Verification items for the finished model (mm, model axes). A direction names the side the tool comes from. Round coordinates to 2 decimals unless told otherwise and drop trailing zeros. Write each loop counter-clockwise with the first axis right and the second up, starting at its lowest first coordinate (ties: lowest second). Pieces come first, ordered by that corner, then holes. Notation, with made-up numbers: (18.5, 61.5) - (42.5, 61.5) arc R14 ccw to (42.5, 86.5) - close; hole circle Ø2 at (55.5, -22.5). An arc over 180 degrees is marked (long way). Write each question's results on one line, items separated by ' | '.
```python
from build123d import *

# Parameters (mm, degrees)
SKETCH_1_W           = 113
SKETCH_1_H           = 113
EXTRUDE_1_DEPTH      = 3
CUT_EXTRUDE_1_REACH  = 161.834
SKETCH_2_R           = 1.7
SKETCH_3_W           = 90
SKETCH_3_H           = 105
EXTRUDE_2_DEPTH      = 2
SKETCH_5_R           = 5
EXTRUDE_3_DEPTH      = 3
CUT_EXTRUDE_2_REACH  = 161.834
SKETCH_6_R           = 1.7
CUT_EXTRUDE_3_REACH  = 161.834
SKETCH_7_R           = 1.7
CUT_EXTRUDE_4_REACH  = 161.884
SKETCH_8_R           = 1.7
EXTRUDE_5_DEPTH      = 90
CUT_EXTRUDE_5_DEPTH  = 2
SKETCH_13_W          = 2
SKETCH_13_H          = 12
EXTRUDE_6_DEPTH      = 11.5
CUT_EXTRUDE_6_REACH  = 162.612
SKETCH_14_R          = 1.7
CUT_EXTRUDE_7_REACH  = 164.681
EXTRUDE_7_DEPTH      = 8.5
SKETCH_17_W          = 2
SKETCH_17_H          = 11.5
EXTRUDE_8_DEPTH      = 3
FILLET_1_R           = 1
CUT_EXTRUDE_8_DEPTH  = 163.681089759
SKETCH_20_W          = 113
SKETCH_20_H          = 12.124355653
CUT_EXTRUDE_9_DEPTH  = 1
CHAMFER_1_SIZE       = 1
SKETCH_21_W          = 7
SKETCH_21_H          = 13.5
CUT_EXTRUDE_10_DEPTH = 163.681089759
SKETCH_22_W          = 5
SKETCH_22_H          = 24
CUT_EXTRUDE_11_DEPTH = 163.681089759
SKETCH_23_W          = 2
SKETCH_23_H          = 19.464101615
CUT_EXTRUDE_12_DEPTH = 2
CHAMFER_2_SIZE       = 2
SKETCH_24_W          = 0.692820323
SKETCH_24_H          = 0.4
CUT_EXTRUDE_13_DEPTH = 95.5
SKETCH_25_W          = 0.692820323
SKETCH_25_H          = 0.4
CUT_EXTRUDE_14_DEPTH = 5.5
SKETCH_26_W          = 0.692820323
SKETCH_26_H          = 0.4
CUT_EXTRUDE_15_DEPTH = 7.5
SKETCH_27_W          = 113
SKETCH_27_H          = 105.875644347
CUT_EXTRUDE_16_DEPTH = 163.339889035
SKETCH_29_W          = 10
SKETCH_29_H          = 5
CUT_EXTRUDE_17_DEPTH = 163.185818036
SKETCH_30_W          = 10
SKETCH_30_H          = 2
CUT_EXTRUDE_18_DEPTH = 37
SKETCH_31_W          = 10
SKETCH_31_H          = 27
EXTRUDE_9_DEPTH      = 1


with BuildPart() as part:
    # 草图1 → 凸台-拉伸1 (new body)
    with BuildSketch(Plane(origin=(0, 0, 0), x_dir=(1, 0, 0), z_dir=(0, 1, 0))):
        with Locations((56.5, 56.5)):
            Rectangle(SKETCH_1_W, SKETCH_1_H)
    extrude(amount=EXTRUDE_1_DEPTH)

    # 草图2 → 切除-拉伸1 (cut, up to next)
    with BuildSketch(Plane(origin=(0, 3, 0), x_dir=(1, 0, 0), z_dir=(0, 1, 0)), mode=Mode.PRIVATE) as cut_extrude_1_sk1:
        with Locations(Location((108.5, 69.95, 0), (0, 0, 270))):
            Circle(SKETCH_2_R)
    cut_extrude_1_tool1 = extrude(cut_extrude_1_sk1.sketch, amount=-CUT_EXTRUDE_1_REACH, mode=Mode.PRIVATE) & part.part
    # 草图2 → 切除-拉伸1 (cut, up to next)
    with BuildSketch(Plane(origin=(0, 3, 0), x_dir=(1, 0, 0), z_dir=(0, 1, 0)), mode=Mode.PRIVATE) as cut_extrude_1_sk2:
        with Locations(Location((108.5, 47.45, 0), (0, 0, 270))):
            Circle(SKETCH_2_R)
    cut_extrude_1_tool2 = extrude(cut_extrude_1_sk2.sketch, amount=-CUT_EXTRUDE_1_REACH, mode=Mode.PRIVATE) & part.part
    # 草图2 → 切除-拉伸1 (cut, up to next)
    with BuildSketch(Plane(origin=(0, 3, 0), x_dir=(1, 0, 0), z_dir=(0, 1, 0)), mode=Mode.PRIVATE) as cut_extrude_1_sk3:
        with Locations(Location((106, 30.4, 0), (0, 0, 270))):
            Circle(SKETCH_2_R)
    cut_extrude_1_tool3 = extrude(cut_extrude_1_sk3.sketch, amount=-CUT_EXTRUDE_1_REACH, mode=Mode.PRIVATE) & part.part
    # 草图2 → 切除-拉伸1 (cut, up to next)
    with BuildSketch(Plane(origin=(0, 3, 0), x_dir=(1, 0, 0), z_dir=(0, 1, 0)), mode=Mode.PRIVATE) as cut_extrude_1_sk4:
        with Locations(Location((106, 10.4, 0), (0, 0, 270))):
            Circle(SKETCH_2_R)
    cut_extrude_1_tool4 = extrude(cut_extrude_1_sk4.sketch, amount=-CUT_EXTRUDE_1_REACH, mode=Mode.PRIVATE) & part.part
    add(cut_extrude_1_tool1.solids().sort_by_distance((108.5, 3, -69.95))[0], mode=Mode.SUBTRACT)
    add(cut_extrude_1_tool2.solids().sort_by_distance((108.5, 3, -47.45))[0], mode=Mode.SUBTRACT)
    add(cut_extrude_1_tool3.solids().sort_by_distance((106, 3, -30.4))[0], mode=Mode.SUBTRACT)
    add(cut_extrude_1_tool4.solids().sort_by_distance((106, 3, -10.4))[0], mode=Mode.SUBTRACT)

    # 草图3 → 凸台-拉伸2 (add)
    with BuildSketch(Plane(origin=(0, 0, 0), x_dir=(1, 0, 0), z_dir=(0, 1, 0))):
        with Locations((55.5, 60.5)):
            Rectangle(SKETCH_3_W, SKETCH_3_H)
    extrude(amount=-EXTRUDE_2_DEPTH)

    # 草图5 → 凸台-拉伸3 (add)
    with BuildSketch(Plane.XZ):
        with Locations((79.5, -1)):
            Circle(SKETCH_5_R)
        with Locations((31.5, -1)):
            Circle(SKETCH_5_R)
    extrude(amount=-EXTRUDE_3_DEPTH)

    # 草图6 → 切除-拉伸2 (cut, up to next)
    with BuildSketch(Plane.XZ, mode=Mode.PRIVATE) as cut_extrude_2_sk1:
        with Locations(Location((31.5, -1, 0), (0, 0, 270))):
            Circle(SKETCH_6_R)
    cut_extrude_2_tool1 = extrude(cut_extrude_2_sk1.sketch, amount=-CUT_EXTRUDE_2_REACH, mode=Mode.PRIVATE) & part.part
    # 草图6 → 切除-拉伸2 (cut, up to next)
    with BuildSketch(Plane.XZ, mode=Mode.PRIVATE) as cut_extrude_2_sk2:
        with Locations(Location((79.5, -1, 0), (0, 0, 270))):
            Circle(SKETCH_6_R)
    cut_extrude_2_tool2 = extrude(cut_extrude_2_sk2.sketch, amount=-CUT_EXTRUDE_2_REACH, mode=Mode.PRIVATE) & part.part
    add(cut_extrude_2_tool1.solids().sort_by_distance((31.5, 0, -1))[0], mode=Mode.SUBTRACT)
    add(cut_extrude_2_tool2.solids().sort_by_distance((79.5, 0, -1))[0], mode=Mode.SUBTRACT)

    # 草图7 → 切除-拉伸3 (cut, up to next)
    with BuildSketch(Plane.XZ, mode=Mode.PRIVATE) as cut_extrude_3_sk1:
        with Locations(Location((5, -10.4, 0), (0, 0, 270))):
            Circle(SKETCH_7_R)
    cut_extrude_3_tool1 = extrude(cut_extrude_3_sk1.sketch, amount=-CUT_EXTRUDE_3_REACH, mode=Mode.PRIVATE) & part.part
    # 草图7 → 切除-拉伸3 (cut, up to next)
    with BuildSketch(Plane.XZ, mode=Mode.PRIVATE) as cut_extrude_3_sk2:
        with Locations(Location((5, -30.4, 0), (0, 0, 270))):
            Circle(SKETCH_7_R)
    cut_extrude_3_tool2 = extrude(cut_extrude_3_sk2.sketch, amount=-CUT_EXTRUDE_3_REACH, mode=Mode.PRIVATE) & part.part
    # 草图7 → 切除-拉伸3 (cut, up to next)
    with BuildSketch(Plane.XZ, mode=Mode.PRIVATE) as cut_extrude_3_sk3:
        with Locations(Location((5, -65.4, 0), (0, 0, 270))):
            Circle(SKETCH_7_R)
    cut_extrude_3_tool3 = extrude(cut_extrude_3_sk3.sketch, amount=-CUT_EXTRUDE_3_REACH, mode=Mode.PRIVATE) & part.part
    add(cut_extrude_3_tool1.solids().sort_by_distance((5, 0, -10.4))[0], mode=Mode.SUBTRACT)
    add(cut_extrude_3_tool2.solids().sort_by_distance((5, 0, -30.4))[0], mode=Mode.SUBTRACT)
    add(cut_extrude_3_tool3.solids().sort_by_distance((5, 0, -65.4))[0], mode=Mode.SUBTRACT)

    # 草图8 → 切除-拉伸4 (cut, up to next)
    with BuildSketch(Plane.XZ.offset(2), mode=Mode.PRIVATE) as cut_extrude_4_sk1:
        with Locations(Location((38, -83, 0), (0, 0, 270))):
            Circle(SKETCH_8_R)
    cut_extrude_4_tool1 = extrude(cut_extrude_4_sk1.sketch, amount=-CUT_EXTRUDE_4_REACH, mode=Mode.PRIVATE) & part.part
    # 草图8 → 切除-拉伸4 (cut, up to next)
    with BuildSketch(Plane.XZ.offset(2), mode=Mode.PRIVATE) as cut_extrude_4_sk2:
        with Locations(Location((73, -83, 0), (0, 0, 270))):
            Circle(SKETCH_8_R)
    cut_extrude_4_tool2 = extrude(cut_extrude_4_sk2.sketch, amount=-CUT_EXTRUDE_4_REACH, mode=Mode.PRIVATE) & part.part
    add(cut_extrude_4_tool1.solids().sort_by_distance((38, -2, -83))[0], mode=Mode.SUBTRACT)
    add(cut_extrude_4_tool2.solids().sort_by_distance((73, -2, -83))[0], mode=Mode.SUBTRACT)

    # 草图10 → 凸台-拉伸5 (add)
    with BuildSketch(Plane(origin=(100.5, 0, 0), x_dir=(0, 0, -1), z_dir=(1, 0, 0))):
        Polygon((113, 0), (116.464101615, -2), (113, -2), align=None)
    extrude(amount=-EXTRUDE_5_DEPTH)

    # 草图11 → 切除-拉伸5 (cut)
    with BuildSketch(Plane(origin=(0, -2, 0), x_dir=(1, 0, 0), z_dir=(0, 1, 0))):
        with BuildLine():
            Line((33, 83), (33, 53))
            ThreePointArc((33, 53), (38, 48), (43, 53))
            Line((43, 53), (43, 83))
            ThreePointArc((43, 83), (38, 88), (33, 83))
        make_face()
        with BuildLine():
            Line((68, 83), (68, 53))
            ThreePointArc((68, 53), (73, 48), (78, 53))
            Line((78, 53), (78, 83))
            ThreePointArc((78, 83), (73, 88), (68, 83))
        make_face()
    extrude(amount=CUT_EXTRUDE_5_DEPTH, mode=Mode.SUBTRACT)

    # 草图13 → 凸台-拉伸6 (add)
    with BuildSketch(Plane.XZ):
        with Locations((4, -83)):
            Rectangle(SKETCH_13_W, SKETCH_13_H)
    extrude(amount=EXTRUDE_6_DEPTH)

    # 草图14 → 切除-拉伸6 (cut, up to next)
    with BuildSketch(Plane.ZY.offset(-3), mode=Mode.PRIVATE) as cut_extrude_6_sk1:
        with Locations((-83.5, -5)):
            Circle(SKETCH_14_R)
    cut_extrude_6_tool1 = extrude(cut_extrude_6_sk1.sketch, amount=-CUT_EXTRUDE_6_REACH, mode=Mode.PRIVATE) & part.part
    add(cut_extrude_6_tool1.solids().sort_by_distance((3, -5, -83.5))[0], mode=Mode.SUBTRACT)

    # 草图15 → 切除-拉伸7 (cut, up to next)
    with BuildSketch(Plane.XZ, mode=Mode.PRIVATE) as cut_extrude_7_sk1:
        Polygon((113, -100.875644347), (106, -113), (113, -113), align=None)
    cut_extrude_7_tool1 = extrude(cut_extrude_7_sk1.sketch, amount=-CUT_EXTRUDE_7_REACH, mode=Mode.PRIVATE) & part.part
    add(cut_extrude_7_tool1.solids().sort_by_distance((110.666667, 0, -108.958548))[0], mode=Mode.SUBTRACT)

    # 草图16 → 凸台-拉伸7 (add)
    with BuildSketch(Plane.XZ):
        Polygon((113, -99.5), (107.5, -99.5), (107.5, -110.401923789), (113, -100.875644347), align=None)
    extrude(amount=EXTRUDE_7_DEPTH)

    # 草图17 → 凸台-拉伸8 (add)
    with BuildSketch(Plane.ZY.offset(-3)):
        with Locations((-78, -5.75)):
            Rectangle(SKETCH_17_W, SKETCH_17_H)
    extrude(amount=EXTRUDE_8_DEPTH)

    # 圆角1
    fillet_1_edges = [part.edges().sort_by_distance(p)[0] for p in [
        (3, -5.75, -79),
    ]]
    fillet(fillet_1_edges, radius=FILLET_1_R)

    # 草图19 → 切除-拉伸8 (cut, through all)
    with BuildSketch(Plane.ZY):
        Polygon((-113, 0), (-107.803847577, 3), (-113, 3), align=None)
    extrude(amount=-CUT_EXTRUDE_8_DEPTH, mode=Mode.SUBTRACT)

    # 草图20 → 切除-拉伸9 (cut)
    with BuildSketch(Plane(origin=(0, 3, 0), x_dir=(1, 0, 0), z_dir=(0, 1, 0))):
        with Locations((56.5, 106.937822173)):
            Rectangle(SKETCH_20_W, SKETCH_20_H)
    extrude(amount=-CUT_EXTRUDE_9_DEPTH, mode=Mode.SUBTRACT)

    # 倒角1
    chamfer_1_edges = [part.edges().sort_by_distance(p)[0] for p in [
        (56.5, 2, -100.875644347),
    ]]
    chamfer(chamfer_1_edges, length=CHAMFER_1_SIZE - 0.0001)  # a hair under: the kernel refuses the full size

    # 草图21 → 切除-拉伸10 (cut, through all)
    with BuildSketch(Plane.XZ.offset(8.5)):
        with Locations((109.5, -106.25)):
            Rectangle(SKETCH_21_W, SKETCH_21_H)
    extrude(amount=-CUT_EXTRUDE_10_DEPTH, mode=Mode.SUBTRACT)

    # 草图22 → 切除-拉伸11 (cut, through all)
    with BuildSketch(Plane.XZ):
        with Locations((2.5, -101)):
            Rectangle(SKETCH_22_W, SKETCH_22_H)
    extrude(amount=-CUT_EXTRUDE_11_DEPTH, mode=Mode.SUBTRACT)

    # 草图23 → 切除-拉伸12 (cut)
    with BuildSketch(Plane.XZ.offset(2)):
        with Locations((11.5, -106.732050808)):
            Rectangle(SKETCH_23_W, SKETCH_23_H)
    extrude(amount=-CUT_EXTRUDE_12_DEPTH, mode=Mode.SUBTRACT)

    # 倒角2
    chamfer_2_edges = [part.edges().sort_by_distance(p)[0] for p in [
        (10.5, -1, -97),
    ]]
    chamfer(chamfer_2_edges, length=CHAMFER_2_SIZE - 0.0001)  # a hair under: the kernel refuses the full size

    # 草图24 → 切除-拉伸13 (cut)
    with BuildSketch(Plane(origin=(100.5, 0, 0), x_dir=(0, 0, -1), z_dir=(1, 0, 0))):
        with Locations((116.117691454, -1.8)):
            Rectangle(SKETCH_24_W, SKETCH_24_H)
    extrude(amount=-CUT_EXTRUDE_13_DEPTH, mode=Mode.SUBTRACT)

    # 草图25 → 切除-拉伸14 (cut)
    with BuildSketch(Plane(origin=(106, 0, 0), x_dir=(0, 0, -1), z_dir=(1, 0, 0))):
        with Locations((112.653589839, 0.2)):
            Rectangle(SKETCH_25_W, SKETCH_25_H)
    extrude(amount=-CUT_EXTRUDE_14_DEPTH, mode=Mode.SUBTRACT)

    # 草图26 → 切除-拉伸15 (cut)
    with BuildSketch(Plane.ZY.offset(-5)):
        with Locations((-112.653589839, 0.2)):
            Rectangle(SKETCH_26_W, SKETCH_26_H)
    extrude(amount=-CUT_EXTRUDE_15_DEPTH, mode=Mode.SUBTRACT)

    # 草图27 → 切除-拉伸16 (cut, through all)
    with BuildSketch(Plane(origin=(0, 2, 0), x_dir=(1, 0, 0), z_dir=(0, 1, 0))):
        with Locations((56.5, 48.937822174)):
            Rectangle(SKETCH_27_W, SKETCH_27_H)
    extrude(amount=CUT_EXTRUDE_16_DEPTH, mode=Mode.SUBTRACT)

    # 草图29 → 切除-拉伸17 (cut, through all)
    with BuildSketch(Plane.XZ):
        with Locations((38, -50.5)):
            Rectangle(SKETCH_29_W, SKETCH_29_H)
        with Locations((73, -50.5)):
            Rectangle(SKETCH_29_W, SKETCH_29_H)
    extrude(amount=CUT_EXTRUDE_17_DEPTH, mode=Mode.SUBTRACT)

    # 草图30 → 切除-拉伸18 (cut)
    with BuildSketch(Plane(origin=(0, 0, -48), x_dir=(-1, 0, 0), z_dir=(0, 0, -1))):
        with Locations((-38, -1)):
            Rectangle(SKETCH_30_W, SKETCH_30_H)
        with Locations((-73, -1)):
            Rectangle(SKETCH_30_W, SKETCH_30_H)
    extrude(amount=-CUT_EXTRUDE_18_DEPTH, mode=Mode.SUBTRACT)

    # 草图31 → 凸台-拉伸9 (add)
    with BuildSketch(Plane.XZ):
        with Locations((38, -24.5)):
            Rectangle(SKETCH_31_W, SKETCH_31_H)
        with Locations((73, -24.5)):
            Rectangle(SKETCH_31_W, SKETCH_31_H)
    extrude(amount=EXTRUDE_9_DEPTH)


solid = part.part
```
(1) Go/stop test with flat-tipped pins: pin 1 Ø1 at (x, z) = (51.5, -14) entering from -Y; pin 2 Ø5.5 at (x, z) = (31.5, -1) entering from +Y; pin 3 Ø0.6 at (y, z) = (-1, -43.5) entering from +X; pin 4 Ø1.9 at (y, z) = (-1.5, -109.5) entering from -X. Record where each tip stops, or that it passes through.
Answer:
pin 1: y = -2 | pin 2: y = 2 | pin 3: x = 100.5 | pin 4: x = 12.5
(2) Section check A-A (z = -47.45). Record the cut outline in (x, y).
Answer:
outline: (0, 0) - (10.5, 0) - (10.5, -2) - (33, -2) - (33, 0) - (43, 0) - (43, -2) - (68, -2) - (68, 0) - (78, 0) - (78, -2) - (100.5, -2) - (100.5, 0) - (106.8, 0) - (106.8, 2) - (0, 2) - close; (110.2, 0) - (113, 0) - (113, 2) - (110.2, 2) - close
(3) Mould release check, pull along Y, two halves, no side actions. Record for faces 1 (the cylindrical face through (77.84, 0.99, -0.63)), 2 (the cylindrical face through (3.99, -4.93, -85.2)), 3 (the flat face through (56, -2, -63)): released by +Y, released by -Y, zero draft, split by the parting line, or undercut.
Answer:
face 1: zero draft | face 2: undercut | face 3: released by -Y
(4) Section check D-D (x = 98). Record the cut outline in (y, z).
Answer:
outline: (-2, -115.77) - (-1.6, -115.77) - (2, -109.54) - (2, 0) - (0, 0) - (0, -8) - (-2, -8) - close
(5) Section check B-B (x = 79.5). Record the cut outline in (y, z).
Answer:
outline: (-2, -115.77) - (-1.6, -115.77) - (2, -109.54) - (2, -2.7) - (0, -2.7) - (0, -8) - (-2, -8) - close; (0, 0.7) - (2, 0.7) - (2, 4) - (0, 4) - close
(6) Section check C-C (y = -5). Record the cut outline in (x, z), plus the area to 3 significant figures.
Answer:
outline: (0, -79) - (2, -79) arc R1 cw to (3, -80) - (3, -81.8) - (5, -81.8) - (5, -77) - (0, -77) - close; (3, -89) - (5, -89) - (5, -85.2) - (3, -85.2) - close | area: 23.4 mm2
(7) Thickness scan on L1, parallel to X at y = 1.3, z = -30.4; L2, parallel to X at y = 0.5, z = -83; L3, parallel to Y at x = 4.55, z = -83.5. Record the ranges inside material, lowest first.
Answer:
L1: 0 to 3.3, 6.7 to 104.3, 107.7 to 113 | L2: 0 to 36.3, 39.7 to 71.3, 74.7 to 113 | L3: -11.5 to -6.7, -3.3 to 2
(8) Set-up check for faces 4 (the flat face through (3, -6, -77)), 5 (the cylindrical face through (73, -1, -88)), 6 (the flat face through (1, 0, -84)), 7 (the flat face through (4, -5, -89)): record each of +Z, -Z, +X, -X, +Y, -Y from which the full face is reachable in a straight line by a thin tool's end or side.
Answer:
face 4: +Z, -X, -Y | face 5: -Y | face 6: -Z, -X, -Y | face 7: -Z, -X, +Y, -Y
